Can you work these out from the model? Positions are in its coordinate system, mm. A direction names the side the tool comes from. Give positions to 0.01 mm unless a question says otherwise; leave off trailing zeros. Order: outer loops, then holes, each group sorted by start corner. A loop starts at its lowest first (then second) coordinate and runs counter-clockwise, first axis right, second up.
```python
from build123d import *

# Parameters (mm, degrees)
BOX_W           = 68
BOX_H           = 60
BOX_DEPTH       = 70
SKETCH_R        = 1.51
POCKET_DEPTH    = 35
SKETCH001_W     = 65
SKETCH001_H     = 2.5
POCKET001_DEPTH = 2
SKETCH002_W     = 60
SKETCH002_H     = 17
POCKET002_DEPTH = 40
SKETCH003_W     = 38
SKETCH003_H     = 9.413655
POCKET003_DEPTH = 47
SKETCH004_R     = 1.51
POCKET004_DEPTH = 68.001
POCKET005_DEPTH = 68.001
SKETCH006_R     = 1.51
POCKET006_DEPTH = 10
PAD_DEPTH       = 10
CHAMFER001_SIZE = 5.5
SKETCH008_R     = 1.5
POCKET007_DEPTH = 68.001
SKETCH009_W     = 59.42001
SKETCH009_H     = 0.5
SKETCH009_W_2   = 59.338872
PAD001_DEPTH    = 35
SKETCH010_W     = 37.356884
SKETCH010_H     = 0.551608
PAD002_DEPTH    = 47
SKETCH011_R     = 1.5
POCKET008_DEPTH = 10
SKETCH012_R     = 1.51
PAD003_DEPTH    = 1


with BuildPart() as part:
    # Box → Box (new body)
    with BuildSketch(Plane(origin=(0, -2, 0), x_dir=(1, 0, 0), z_dir=(0, 0, 1))):
        with Locations((34, 30)):
            Rectangle(BOX_W, BOX_H)
    extrude(amount=BOX_DEPTH)


with BuildPart() as part_1:
    # BaseFeature placement: moved
    add(part.part.moved(Location((0, 2, 0))))

    # Sketch (on Face6 of BaseFeature) → Pocket (cut)
    with BuildSketch(Plane.XY.offset(70)):
        with Locations((20, 15)):
            Circle(SKETCH_R)
        with Locations((48, 15)):
            Circle(SKETCH_R)
        Polygon((1.5, 55.5), (66.5, 55.5), (66.5, 58), (64, 58), (64, 62.74518), (4, 62.74518), (4, 58), (1.5, 58), align=None)
    extrude(amount=-POCKET_DEPTH, mode=Mode.SUBTRACT)

    # Sketch001 (on Face16 of Pocket) → Pocket001 (cut)
    with BuildSketch(Plane.XY.offset(35)):
        with Locations((34, 56.75)):
            Rectangle(SKETCH001_W, SKETCH001_H)
    extrude(amount=-POCKET001_DEPTH, mode=Mode.SUBTRACT)

    # Sketch002 (on Face3 of Pocket001) → Pocket002 (cut)
    with BuildSketch(Plane.XY.offset(70)):
        with Locations((34, 40.5)):
            Rectangle(SKETCH002_W, SKETCH002_H)
    extrude(amount=-POCKET002_DEPTH, mode=Mode.SUBTRACT)

    # Sketch003 (on Face3 of Pocket002) → Pocket003 (cut)
    with BuildSketch(Plane.XY.offset(70)):
        with Locations((34, -0.162125)):
            Rectangle(SKETCH003_W, SKETCH003_H)
    extrude(amount=-POCKET003_DEPTH, mode=Mode.SUBTRACT)

    # Sketch004 (on Face1 of Pocket003) → Pocket004 (cut, through all)
    with BuildSketch(Plane(origin=(0, 0, 0), x_dir=(0, -1, 0), z_dir=(-1, 0, 0))):
        with Locations((-37.5, 21)):
            Circle(SKETCH004_R)
        with Locations((-2.5, 21)):
            Circle(SKETCH004_R)
    extrude(amount=-POCKET004_DEPTH, mode=Mode.SUBTRACT)

    # Sketch005 (on Face8 of Pocket004) → Pocket005 (cut, through all)
    with BuildSketch(Plane.YZ.offset(68)):
        Polygon((25.567, -11.191082), (76.135516, -11.191082), (76.135516, 10.70104), (43.079702, 10.70104), align=None)
    extrude(amount=-POCKET005_DEPTH, mode=Mode.SUBTRACT)

    # Sketch006 (on Face4 of Pocket005) → Pocket006 (cut)
    with BuildSketch(Plane(origin=(0, 0, 10.70104), x_dir=(1, 0, 0), z_dir=(0, 0, -1))):
        with Locations((19, -55.82514)):
            Circle(SKETCH006_R)
        with Locations((49, -55.82514)):
            Circle(SKETCH006_R)
    extrude(amount=-POCKET006_DEPTH, mode=Mode.SUBTRACT)

    # Sketch007 (on Face4 of Pocket006) → Pad (join)
    with BuildSketch(Plane(origin=(0, 0, 10.70104), x_dir=(1, 0, 0), z_dir=(0, 0, -1))):
        with BuildLine():
            ThreePointArc((11.5, -60), (34, -65.600118), (56.5, -60))
            Line((54.883537, -58.581185), (56.5, -60))
            Line((13.061421, -58.581185), (54.883537, -58.581185))
            Line((11.5, -60), (13.061421, -58.581185))
        make_face()
    extrude(amount=-PAD_DEPTH)

    # Chamfer001
    chamfer001_edges = [part_1.edges().sort_by_distance(p)[0] for p in [
        (34, 60, 20.70104),
    ]]
    chamfer(chamfer001_edges, length=CHAMFER001_SIZE)

    # Sketch008 (on Face8 of Chamfer001) → Pocket007 (cut, through all)
    with BuildSketch(Plane(origin=(0, 0, 0), x_dir=(0, -1, 0), z_dir=(-1, 0, 0))):
        with Locations((-44.590099, 65.813534)):
            Circle(SKETCH008_R)
        with Locations((-10.543741, 65.813534)):
            Circle(SKETCH008_R)
    extrude(amount=-POCKET007_DEPTH, mode=Mode.SUBTRACT)

    # Sketch009 (on Face1 of ReferenceChamfer002001) → Pad001 (join)
    with BuildSketch(Plane.XY.offset(35)):
        with Locations((34.071956, 59.544491)):
            Rectangle(SKETCH009_W, SKETCH009_H)
        with Locations((34.120748, 58.559672)):
            Rectangle(SKETCH009_W_2, SKETCH009_H)
    extrude(amount=PAD001_DEPTH)

    # Sketch010 (on Face49 of Pad001) → Pad002 (join)
    with BuildSketch(Plane.XY.offset(23)):
        with Locations((34.035056, 0.529754)):
            Rectangle(SKETCH010_W, SKETCH010_H)
    extrude(amount=PAD002_DEPTH)

    # Sketch011 (on Face17 of Pad002) → Pocket008 (cut)
    with BuildSketch(Plane.XZ):
        with Locations((6, 25.127343)):
            Circle(SKETCH011_R)
        with Locations((62, 25.127343)):
            Circle(SKETCH011_R)
    extrude(amount=-POCKET008_DEPTH, mode=Mode.SUBTRACT)

    # Sketch012 (on Face17 of Pocket008) → Pad003 (join)
    with BuildSketch(Plane.XZ):
        Polygon((0, 33), (15, 33), (15, 23), (53, 23), (53, 33), (68, 33), (68, 13.022348), (0, 13.022348), align=None)
        with Locations((6, 25.127343)):
            Circle(SKETCH012_R, mode=Mode.SUBTRACT)
        with Locations((62, 25.127343)):
            Circle(SKETCH012_R, mode=Mode.SUBTRACT)
    extrude(amount=PAD003_DEPTH)


solid = part_1.part
```
1) Suppose I cut it at B-B (y = 15). Please give me the cut outline in (x, z).
2) Suppose I cut it at C-C (y = 2.5). Please give me the cut outline in (x, z), and give its area (3 significant figures).
3) Which directions (+Z, -Z, +X, -X, +Y, -Y) give clear straight access to the entire face, cutting with the end or side of a thin tool? Please do faces 1 (the face through (15, 2, 47)), 2 (the face through (34, 41, 30)), 3 (the face through (4, 59, 53)), 4 (the face through (60.89, -0.49, 26.15)).
4) We'd pull the mould along Y, two halves only. Please class faces 5 (the face through (34.476, 38.859, 5.425)), 6 (the face through (68, 30, 35)), 7 (the face through (33.524, 36.105, 20.422)): +Y half, -Y half, draft (parallel to the pull), parting line (faces both ways), or undercut.
5) If I drill on line 1 (Y direction, x = 4.5, z = 61); line 2 (Y direction, x = 37.5, z = 38); line 3 (Z direction, x = 62, y = 5.5), over which ranges is the centre line in solid material (lowest first)?
6) Suppose I cut it at A-A (z = 40.5). Give the number of separate pieces and of enclosed holes in the cut face, and give its area (3 significant figures).
7) I'm going to push flat-ended pins straight in: pin 1 Ø7 at (x, y) = (19, 58.5) entering from -Z; pin 2 Ø1.5 at (x, z) = (61.5, 25) entering from -Y; pin 3 Ø4 at (x, z) = (42, 49) entering from +Y. Where does each tip first touch, or does it pass through?
8) Suppose I cut it at D-D (z = 15). Please give me the cut outline in (x, y).
Results:
1. outline: (0, 0) - (68, 0) - (68, 70) - (49.51, 70) - (49.51, 35) - (46.49, 35) - (46.49, 70) - (21.51, 70) - (21.51, 35) - (18.49, 35) - (18.49, 70) - (0, 70) - close
2. outline: (0, 0) - (68, 0) - (68, 19.49) - (0, 19.49) - close; (0, 22.51) - (68, 22.51) - (68, 70) - (53, 70) - (53, 23) - (15, 23) - (15, 70) - (0, 70) - close; hole circle Ø3 at (6, 25.13); hole circle Ø3 at (62, 25.13)
2. area: 2,750 mm2
3. face 1: +Z, -Y
3. face 2: +Z
3. face 3: +Z, +Y
3. face 4: -Y
4. face 5: +Y half
4. face 6: draft
4. face 7: undercut
5. line 1: y = 0 to 32, 49 to 55.5, 58.31 to 58.81, 59.29 to 59.79
5. line 2: y = 0.25 to 0.81, 4.54 to 32, 49 to 55.5, 58.31 to 58.81, 59.29 to 59.79
5. line 3: z = 0 to 23.63, 26.63 to 70
6. separate pieces: 4
6. enclosed holes: 3
6. area: 2,670 mm2
7. pin 1: stops at z = 10.7
7. pin 2: stops at y = 10
7. pin 3: stops at y = 59.79
8. outline: (0, -1) - (68, -1) - (68, 60) - (56.5, 60) arc R48 ccw to (11.5, 60) - (0, 60) - close; hole circle Ø3.02 at (19, 55.83); hole circle Ø3.02 at (49, 55.83)
